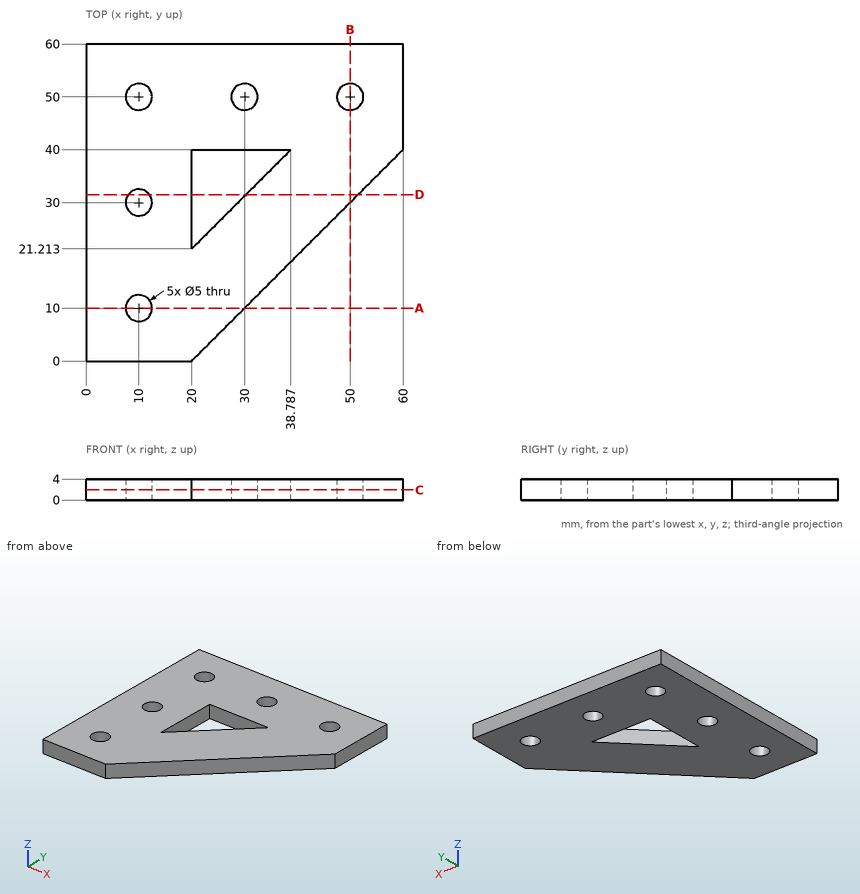
Job drawing, mm, ordinate dimensions from the low corner. One solid piece. Coordinates: 2 decimals unless noted, no trailing zeros. Order: outer loops, then holes, each group sorted by start corner. A loop starts at its lowest first (then second) coordinate and runs counter-clockwise, first axis right, second up. Notation, with made-up numbers: (36.25, 75.25) -> (44.25, 75.25) arc R22 cw to (44.25, 86.25) -> close; hole circle Ø9 at (20.25, 79). An arc over 180 degrees is marked (long way). Answer in a Markdown table with one row per item. Add a question column.
Q1. Wall check: line 1 along Y through (x, z) = (10, 1.4); line 2 along X through (y, z) = (32, 1.2); line 3 along Y through (x, z) = (30, 0.65). Give the ranges that are in metal, low to high. Write a range as [from, to].
Q2. Band-saw the part on C-C, the plane z = 1.95. List the corners of the cut face in (x, y), then the cut area to 3 significant figures.
Q3. Band-saw the part on B-B, the plane x = 50. List the corners of the cut face in (y, z), then the cut area to 3 significant figures.
Q4. Band-saw the part on D-D, the plane y = 31.5. List the corners of the cut face in (x, z).
Q5. Band-saw the part on A-A, the plane y = 10. List the corners of the cut face in (x, z), then the cut area to 3 significant figures.
Answers follow:
| question | item | result |
|---|---|---|
| 1 | line 1 | [0, 7.5], [12.5, 27.5], [32.5, 47.5], [52.5, 60] |
| 1 | line 2 | [0, 8.5], [11.5, 20], [30.79, 52] |
| 1 | line 3 | [10, 31.21], [40, 47.5], [52.5, 60] |
| 2 | outline | (0, 0) -> (20, 0) -> (60, 40) -> (60, 60) -> (0, 60) -> close; hole circle Ø5 at (10, 10); hole circle Ø5 at (10, 30); hole circle Ø5 at (10, 50); hole (20, 21.21) -> (38.79, 40) -> (20, 40) -> close; hole circle Ø5 at (30, 50); hole circle Ø5 at (50, 50) |
| 2 | area | 2,530 mm^2 |
| 3 | outline | (30, 0) -> (47.5, 0) -> (47.5, 4) -> (30, 4) -> close; (52.5, 0) -> (60, 0) -> (60, 4) -> (52.5, 4) -> close |
| 3 | area | 100 mm^2 |
| 4 | outline | (0, 0) -> (8, 0) -> (8, 4) -> (0, 4) -> close; (12, 0) -> (20, 0) -> (20, 4) -> (12, 4) -> close; (30.29, 0) -> (51.5, 0) -> (51.5, 4) -> (30.29, 4) -> close |
| 5 | outline | (0, 0) -> (7.5, 0) -> (7.5, 4) -> (0, 4) -> close; (12.5, 0) -> (30, 0) -> (30, 4) -> (12.5, 4) -> close |
| 5 | area | 100 mm^2 |
